```python
from build123d import *

# Parameters (mm, degrees)
F2_R     = 5.5499
F3_DEPTH = 31.878
F4_SIZE  = 1.524
F5_R     = 1.524


with BuildPart() as f1:
    # F0 (on Front) → F1 (revolve)
    with BuildSketch(Plane.XZ):
        with BuildLine():
            Line((-50.80635, 0), (0, 0))
            Line((0, 0), (0, 27.94))
            Line((0, 27.94), (-28.83281, 27.94))
            ThreePointArc((-28.83281, 27.94), (-29.371625, 28.163185), (-29.59481, 28.702))
            Line((-29.59481, 28.702), (-29.59481, 29.464))
            Line((-29.59481, 29.464), (-30.05074, 29.464))
            ThreePointArc((-30.05074, 29.464), (-30.481792, 29.642548), (-30.66034, 30.0736))
            Line((-30.66034, 30.0736), (-30.66034, 31.115))
            ThreePointArc((-30.66034, 31.115), (-30.883525, 31.653815), (-31.42234, 31.877))
            Line((-31.42234, 31.877), (-47.50435, 31.877))
            Line((-47.50435, 31.877), (-50.67935, 28.702))
            Line((-50.67935, 28.702), (-50.67935, 12.7))
            Line((-50.67935, 12.7), (-50.80635, 12.7))
            Line((-50.80635, 12.7), (-50.80635, 0))
        make_face()
    revolve(axis=Axis((0, 0, 13.97), (0, 0, -1)))

    # F2 (on Top) → F3 (cut, through all)
    with BuildSketch(Plane.XY):
        Circle(F2_R)
    extrude(amount=F3_DEPTH, mode=Mode.SUBTRACT)

    # F4
    f4_edges = [f1.edges().sort_by_distance(p)[0] for p in [
        (-5.5499, 0, 27.94),
        (-5.5499, 0, 0),
    ]]
    chamfer(f4_edges, length=F4_SIZE)

    # F5
    f5_edges = [f1.edges().sort_by_distance(p)[0] for p in [
        (50.80635, 0, 0),
    ]]
    fillet(f5_edges, radius=F5_R)


solid = f1.part
```
For this review, take the finished solid that the model builds, in its own axes (mm). A direction names the side the tool comes from. Coordinates: 2 decimals unless noted, no trailing zeros. Order: outer loops, then holes, each group sorted by start corner. A loop starts at its lowest first (then second) coordinate and runs counter-clockwise, first axis right, second up. Notation, with made-up numbers: (0.5, -4) - (8.5, -4) arc R23 ccw to (8.5, 24) - close; hole circle Ø9 at (-8.5, 27). An arc over 180 degrees is marked (long way). Answer as a JSON object with one key per item and string values. Group by question number.
1. We need section C-C on z = 20.5. State the section outline as (x, y) points, then the cut area to 3 significant figures.
2. For probe 1 along Y at (x, z) = (0, 14); probe 2 along X at (y, z) = (0.5, 2); probe 3 along Z at (x, y) = (-20, -8.5), list the stretches that pass through material, from the lowest coordinate up.
3. We need section D-D on z = 8. State the section outline as (x, y) points.
4. The part is to be moulded in two halves that separate along X. For faces 1 (the cylindrical face through (5.127, -2.126, 13.796)), 2 (the conical face through (-45.5, 14.33, 31.68)), 3 (the flat face through (-10, 1, 0)), say which applies: pulls with the +X half, pulls with the -X half, needs draft (parallel to the pull), parting line crosses it, or undercut.
5. For faces 4 (the cylindrical face through (6.42, -28.89, 29.09)), 5 (the cylindrical face through (-23.444, -45.074, 7.034)), list the 3-axis set-ups (+Z, -Z, +X, -X, +Y, -Y) from which the entire face can be reached by the end or side of a thin tool; tool diameter is ignored.
6. Clearance check with flat-ended pins moving along their axes: P1, Ø10, axis at x = -36, z = 8, coming from the +Y side; P2, Ø12, axis at y = -35, z = 7, coming from the -X side; P3, Ø2, axis at x = 25, z = 11, coming from the +Y side. State where each tip first meets the part, or that it passes through.
Final values:
{
 "1": {"outline": "circle Ø101.36 at (0, 0); hole circle Ø11.1 at (0, 0)", "area": "7,970 mm²"},
 "2": {"probe 1": "-50.68 to -5.55, 5.55 to 50.68", "probe 2": "-50.8 to -5.53, 5.53 to 50.8", "probe 3": "0 to 27.94"},
 "3": {"outline": "circle Ø101.61 at (0, 0); hole circle Ø11.1 at (0, 0)"},
 "4": {"face 1": "undercut", "face 2": "parting line crosses it", "face 3": "needs draft"},
 "5": {"face 4": "+Z", "face 5": "+Z, -Z"},
 "6": {"P1": "y = 40.25", "P2": "x = -41.72", "P3": "y = 44.78"}
}
